Verification items for the finished model (mm, model axes). Round coordinates to 2 decimals unless told otherwise and drop trailing zeros. Loops run counter-clockwise (first coordinate to the right, second up) from the corner with the lowest first, then second, coordinate; pieces in that order, holes last. Notation, with made-up numbers: (-11, -31.5) - (38, -31.5) arc R33 cw to (38, 2.5) - close; hole circle Ø4 at (59, -20.5). An arc over 180 degrees is marked (long way). Use a Markdown table: item, result. Add a question column.
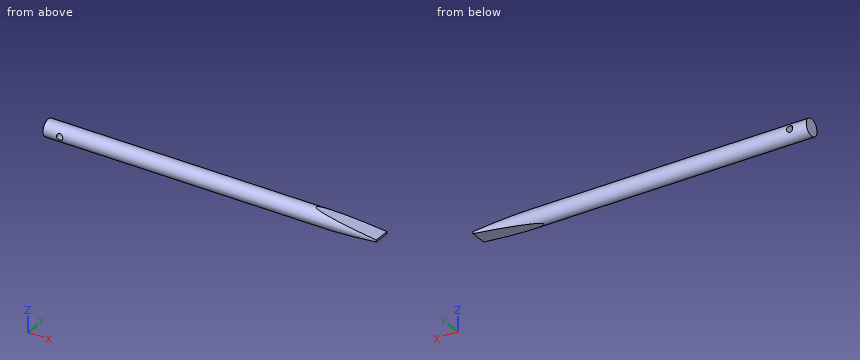
```python
from build123d import *

# Parameters (mm, degrees)
F0_R          = 3.175
F1_DEPTH      = 127
F3_DEPTH      = 25.4
F3_DEPTH_BACK = 25.4
F4_R          = 1.1938
F6_DEPTH      = 3.175
F6_DEPTH_BACK = 3.175


# Not quite as in the source:
# - the program builds the solid bodies; features that only make, move or delete a surface that nothing else refers to are left out


with BuildPart() as f1:
    # F0 (on Right) → F1 (new body)
    with BuildSketch(Plane.YZ):
        Circle(F0_R)
    extrude(amount=-F1_DEPTH)

    # F2 (on Front) → F3 (cut, two sides)
    with BuildSketch(Plane.XZ) as f3_sk:
        Polygon((-25.4, 3.2325035427), (0, 0.381), (0, 3.2325035427), align=None)
        Polygon((0, -3.2135259826), (0, -0.381), (-25.4, -3.2325035427), align=None)
    extrude(amount=-F3_DEPTH, mode=Mode.SUBTRACT)
    extrude(f3_sk.sketch, amount=F3_DEPTH_BACK, mode=Mode.SUBTRACT)

    # F4 (on Front) → F6 (cut, two sides)
    with BuildSketch(Plane.XZ) as f6_sk:
        with Locations((-120.65, 0)):
            Circle(F4_R)
    extrude(amount=F6_DEPTH, mode=Mode.SUBTRACT)
    extrude(f6_sk.sketch, amount=-F6_DEPTH_BACK, mode=Mode.SUBTRACT)


solid = f1.part
```
Q1. Section check B-B on x = -120.65. Record the cut outline in (y, z) (3 decimals).
Q2. Section check C-C on x = -56. Record the cut outline in (y, z) (3 decimals), plus the area to 3 significant figures.
Q3. Section check D-D on x = -15. Record the cut outline in (y, z) (3 decimals), plus the area to 3 significant figures.
Q4. Section check A-A on y = 1.5. Record the cut outline in (x, z).
Q5. Thickness scan on line 1 along X through (y, z) = (-1.6, 0); line 2 along Z through (x, y) = (-120.65, -1.65); line 3 along Z through (x, y) = (-32.5, 0.25). Record the ranges inside material, lowest first.
Q6. Go/stop test with a flat-tipped pin: pin 1 Ø1.4 at (x, z) = (-120.65, 0) entering from -Y. Record where the tip stops, or that it passes through.
Determined:
| question | item | result |
|---|---|---|
| 1 | outline | (-2.942, -1.194) arc R3.175 ccw to (2.942, -1.194) - close; (-2.942, 1.194) - (2.942, 1.194) arc R3.175 ccw to start |
| 2 | outline | circle Ø6.35 at (0, 0) |
| 2 | area | 31.7 mm² |
| 3 | outline | (-2.412, -2.065) - (2.412, -2.065) arc R3.175 ccw to (2.412, 2.065) - (-2.412, 2.065) arc R3.175 ccw to start |
| 3 | area | 24.2 mm² |
| 4 | outline | (-127, -2.8) - (-21.53, -2.8) - (0, -0.38) - (0, 0.38) - (-21.53, 2.8) - (-127, 2.8) - close; hole circle Ø2.39 at (-120.65, 0) |
| 5 | line 1 | x = -127 to -121.84, -119.46 to 0 |
| 5 | line 2 | z = -2.71 to -1.19, 1.19 to 2.71 |
| 5 | line 3 | z = -3.17 to 3.17 |
| 6 | pin 1 | passes through |
